```python
from build123d import *

# Parameters (mm, degrees)
F1_W       = 7.2
F1_H       = 6.41
F2_DEPTH   = 2.9
F3_W       = 4.6
F3_H       = 6.41
F4_DEPTH   = 0.955
F5_DEPTH   = 3.955
F6_R       = 0.2
F7_R       = 0.79
F8_DEPTH   = 4
F9_SIZE2   = 0.7
F9_SIZE    = 1.2124355653
F9_2_SIZE2 = 0.7
F9_2_SIZE  = 1.2124355653
F11_DEPTH  = 12.5


# Not quite as in the source:
# - a feature names something its author has since deleted; it is built from what else it names


with BuildPart() as f2:
    # F1 (on face) → F2 (new body)
    with BuildSketch(Plane.XY):
        with Locations((1.1224337457, -1.1278976017)):
            Rectangle(F1_W, F1_H)
    extrude(amount=F2_DEPTH)

    # F3 (on face) → F4 (join)
    with BuildSketch(Plane.XY.offset(2.9)):
        with Locations((-0.1775662543, -1.1278976017)):
            Rectangle(F3_W, F3_H)
    extrude(amount=F4_DEPTH)

    # F3 (on face) → F5 (join)
    with BuildSketch(Plane.XY.offset(2.9)):
        with Locations((-0.1775662543, -1.1278976017)):
            Rectangle(F3_W, F3_H)
    extrude(amount=-F5_DEPTH)

    # F6
    f6_edges = [f2.edges().sort_by_distance(p)[0] for p in [
        (2.122434, -1.127898, 3.855),
        (-0.177566, -4.332898, 3.855),
        (-2.477566, -1.127898, 3.855),
        (-0.177566, 2.077102, 3.855),
        (3.422434, -4.332898, 2.9),
        (2.122434, -4.332898, 3.3775),
        (-2.477566, -4.332898, 1.4),
        (-0.177566, -4.332898, -1.055),
        (2.122434, -1.127898, -1.055),
        (-0.177566, 2.077102, -1.055),
        (2.122434, -4.332898, -0.5275),
        (3.422434, -4.332898, 0),
        (2.122434, 2.077102, -0.5275),
        (3.422434, 2.077102, 2.9),
        (2.122434, 2.077102, 3.3775),
        (3.422434, 2.077102, 0),
        (-2.477566, 2.077102, 1.4),
        (-2.477566, -1.127898, -1.055),
        (2.122434, -1.127898, 0),
    ]]
    fillet(f6_edges, radius=F6_R)

    # F7 (on face) → F8 (join)
    with BuildSketch(Plane.YZ.offset(4.7224337457)):
        with Locations((-2.7930222052, 1.5)):
            Circle(F7_R)
        with Locations((0.5366023983, 1.45)):
            Circle(F7_R)
    extrude(amount=F8_DEPTH)

    # F9
    f9_edges = [f2.edges().sort_by_distance(p)[0] for p in [
        (8.722434, -3.583022, 1.5),
    ]]
    f9_side = f2.faces().sort_by_distance((6.722434, -3.583022, 1.5))[0]
    chamfer(f9_edges, length=F9_SIZE, length2=F9_SIZE2, reference=f9_side)

    # F9#2
    f9_2_edges = [f2.edges().sort_by_distance(p)[0] for p in [
        (8.722434, -0.253398, 1.45),
    ]]
    f9_2_side = f2.faces().sort_by_distance((6.722434, -0.253398, 1.45))[0]
    chamfer(f9_2_edges, length=F9_2_SIZE, length2=F9_2_SIZE2, reference=f9_2_side)

    # F10 (on face) → F11 (join)
    with BuildSketch(Plane(origin=(-2.4775662543, 0, 0), x_dir=(0, -1, 0), z_dir=(-1, 0, 0))):
        with BuildLine():
            Line((2.6228976017, 3.555), (-0.3771023983, 3.555))
            add(Edge.make_bspline(
                [(-0.3771023983, 3.555), (-0.9371962785, 2.8481079618), (-2.0580811679, 1.3923591855), (-0.9290927555, -0.0252525917), (-0.3671023983, -0.755)],
                knots=[0, 0, 0, 0, 0.4994437063, 1, 1, 1, 1], degree=3))
            Line((-0.3671023983, -0.755), (2.6328976017, -0.755))
            add(Edge.make_bspline(
                [(2.6328976017, -0.755), (3.1901916784, 0.0098145578), (4.3309296415, 1.3596346202), (3.1935954585, 2.8839832867), (2.6228976017, 3.555)],
                knots=[0, 0, 0, 0, 0.5000783208, 1, 1, 1, 1], degree=3))
        make_face()
    extrude(amount=F11_DEPTH)


solid = f2.part
```
For this review, take the finished solid that the model builds, in its own axes (mm). A direction names the side the tool comes from. Coordinates: 2 decimals unless noted, no trailing zeros. Write each loop counter-clockwise with the first axis right and the second up, starting at its lowest first coordinate (ties: lowest second). Pieces come first, ordered by that corner, then holes. Notation, with made-up numbers: (87, 87) - (114, 87) arc R27 cw to (114, 121) - close; hole circle Ø2 at (-29.75, 70). An arc over 180 degrees is marked (long way). Answer in a Markdown table with one row per item. Add a question column.
Q1. We need section A-A, the plane x = 3.5. State the section outline as (y, z) points.
Q2. Draft analysis for pull direction Y (two halves, no side actions). For faces 4 (the flat face through (-9, -1, 3.555)), 5 (the conical face through (8.259, -2.84, 1.854)), 6 (the flat face through (0, 2.077, 1)), state which applies: +Y half, -Y half, draft (parallel to the pull), parting line (faces both ways), or undercut.
Q3. We need section B-B, the plane y = -1.5. State the section outline as (x, z) points (3 decimals).
Q4. For P1, Ø1, axis at x = -6.5, z = 2, coming from the +Y side; P2, Ø3, axis at x = -9, y = -0.5, coming from the -Z side (3 decimals); P3, Ø2.5, axis at x = -6.5, y = -1, coming from the +Z side (3 decimals), all flat-tipped, find the tip position at first contact; note any pin that passes through.
Q5. For probe 1 along Z at (x, y) = (-12.25, -2) (3 decimals); probe 2 along Z at (x, y) = (4.5, 1); probe 3 along X at (y, z) = (-0.25, 0.8), list the stretches that pass through material, from the lowest coordinate up.
Q6. Tool access review of faces 1 (the flat face through (-9, -1, -0.755)), 2 (the cylindrical face through (6.097, 0.961, 2.116)), 3 (the flat face through (4, -1, 0)): name each direction out of +Z, -Z, +X, -X, +Y, -Y from which nothing blocks a thin tool from reaching the whole face with its end or side.
Answer list:
| question | item | result |
|---|---|---|
| 1 | outline | (-4.33, 0.2) arc R0.2 ccw to (-4.13, 0) - (1.88, 0) arc R0.2 ccw to (2.08, 0.2) - (2.08, 2.7) arc R0.2 ccw to (1.88, 2.9) - (-4.13, 2.9) arc R0.2 ccw to (-4.33, 2.7) - close |
| 2 | face 4 | draft |
| 2 | face 5 | undercut |
| 2 | face 6 | +Y half |
| 3 | outline | (-14.978, -0.755) - (-2.478, -0.755) - (-2.478, -0.855) arc R0.2 ccw to (-2.278, -1.055) - (1.922, -1.055) arc R0.2 ccw to (2.122, -0.855) - (2.122, -0.2) arc R0.2 cw to (2.322, 0) - (4.722, 0) - (4.722, 2.9) - (2.122, 2.9) - (2.122, 3.655) arc R0.2 ccw to (1.922, 3.855) - (-2.278, 3.855) arc R0.2 ccw to (-2.478, 3.655) - (-2.478, 3.555) - (-14.978, 3.555) - close |
| 4 | P1 | stops at y = 1.49 |
| 4 | P2 | stops at z = -0.755 |
| 4 | P3 | stops at z = 3.555 |
| 5 | probe 1 | z = -0.755 to 3.555 |
| 5 | probe 2 | z = 0 to 2.9 |
| 5 | probe 3 | x = -14.98 to 4.72 |
| 6 | face 1 | -Z, -X, +Y, -Y |
| 6 | face 2 | +X |
| 6 | face 3 | -Z, +X, +Y, -Y |
